Source: CAD feature listing. Evaluate the final solid. Frame: model axes, mm. Face numbers are marked on the shaded views. A direction names the side the tool comes from. Coordinates: 2 decimals unless noted, no trailing zeros. Order: outer loops, then holes, each group sorted by start corner. A loop starts at its lowest first (then second) coordinate and runs counter-clockwise, first axis right, second up. Notation, with made-up numbers: (-21, 69.25) -> (3, 69.25) arc R36 ccw to (3, 104.25) -> close; hole circle Ø8 at (8.25, 7.25). An arc over 180 degrees is marked (long way). Write item = value, one per line. Start each with the question number.
Item 1: Section query C-C (y = 5.5). Output: boundary loops of the cut face in (x, z).
Item 2: Set-up query: the marked faces 4, 5 and 6. Return all of +Z, -Z, +X, -X, +Y, -Y with unobstructed straight access to the full face (end or side cutting, diameter ignored); none if empty.
Item 3: Ray query, line 1 along X through (y, z) = (0.9, 0); line 2 along Z through (x, y) = (0.25, 4.5); line 3 along X through (y, z) = (1.75, -5.25). Return the intervals inside material, ascending. Write a range as [from, to].
Item 4: Section query B-B (x = -4.5). Output: boundary loops of the cut face in (y, z).
Item 5: Mould query, pull axis X, two halves, no side actions, for the marked faces 1, 2 and 3. Classes: released by +X, released by -X, zero draft, split by the parting line, or undercut.
Item 6: Section query A-A (z = 0). Output: boundary loops of the cut face in (x, y).
Item 7: Section query D-D (z = 4.5). Output: boundary loops of the cut face in (x, y).
Item 8: Contact query for flat-ended pins moving along their axis: pin 1 (1.6 mm diameter, centred on x = -4.5, z = 0, fed in from -Y); pin 2 (6 mm diameter, centred on x = 4, z = 2.5, fed in from +Y); pin 3 (6 mm diameter, centred on x = 5.5, y = 8.5, fed in from -Z). Output: stop coordinate, or through.
```python
from build123d import *

# Parameters (mm, degrees)
SKETCH_1_R          = 7
EXTRUDE_1_DEPTH     = 9
SKETCH_2_R          = 1
CUT_EXTRUDE_2_DEPTH = 2.5
SKETCH_3_R          = 0.5
EXTRUDE_2_DEPTH     = 3.8


with BuildPart() as part:
    # 草图1 → 凸台-拉伸1 (new body)
    with BuildSketch(Plane(origin=(0, 0, 0), x_dir=(1, 0, 0), z_dir=(0, 1, 0))):
        with Locations(Location((0, 0, 0), (0, 0, 270))):
            Circle(SKETCH_1_R)
    extrude(amount=EXTRUDE_1_DEPTH)

    # 草图2 → 切除-拉伸2 (cut)
    with BuildSketch(Plane.XZ):
        with Locations(Location((0, 4.5, 0), (0, 0, 270))):
            Circle(SKETCH_2_R)
        with Locations(Location((0, -4.5, 0), (0, 0, 270))):
            Circle(SKETCH_2_R)
        with Locations(Location((4.5, 0, 0), (0, 0, 270))):
            Circle(SKETCH_2_R)
        with Locations(Location((-4.5, 0, 0), (0, 0, 90))):
            Circle(SKETCH_2_R)
    extrude(amount=-CUT_EXTRUDE_2_DEPTH, mode=Mode.SUBTRACT)

    # 草图3 → 凸台-拉伸2 (add)
    with BuildSketch(Plane(origin=(0, 9, 0), x_dir=(1, 0, 0), z_dir=(0, 1, 0))):
        with Locations(Location((0, 0, 0), (0, 0, 270))):
            Circle(SKETCH_3_R)
    extrude(amount=EXTRUDE_2_DEPTH)


solid = part.part
```
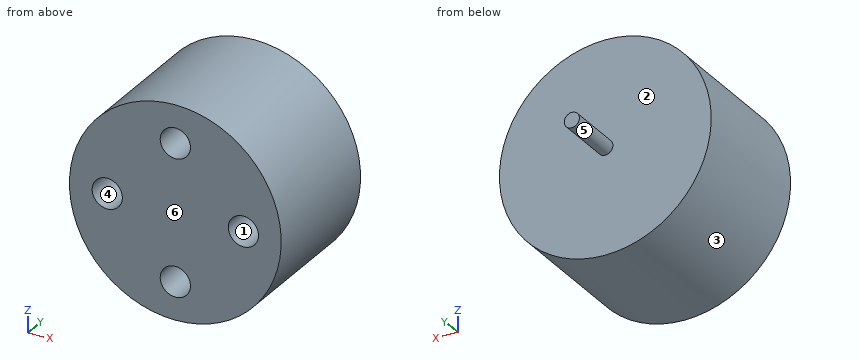
Computed:
q1.outline = circle Ø14 at (0, 0)
q2.face_4 = -Y
q2.face_5 = +Y
q2.face_6 = +Z, -Z, +X, -X, -Y
q3.line_1 = [-7, -5.5], [-3.5, 3.5], [5.5, 7]
q3.line_2 = [-7, 7]
q3.line_3 = [-4.63, -0.66], [0.66, 4.63]
q4.outline = (0, -5.36) -> (9, -5.36) -> (9, 5.36) -> (0, 5.36) -> (0, 1) -> (2.5, 1) -> (2.5, -1) -> (0, -1) -> close
q5.face_1 = undercut
q5.face_2 = zero draft
q5.face_3 = split by the parting line
q6.outline = (-7, 0) -> (-5.5, 0) -> (-5.5, 2.5) -> (-3.5, 2.5) -> (-3.5, 0) -> (3.5, 0) -> (3.5, 2.5) -> (5.5, 2.5) -> (5.5, 0) -> (7, 0) -> (7, 9) -> (0.5, 9) -> (0.5, 12.8) -> (-0.5, 12.8) -> (-0.5, 9) -> (-7, 9) -> close
q7.outline = (-5.36, 0) -> (-1, 0) -> (-1, 2.5) -> (1, 2.5) -> (1, 0) -> (5.36, 0) -> (5.36, 9) -> (-5.36, 9) -> close
q8.pin_1 = 2.5
q8.pin_2 = 9
q8.pin_3 = -6.54
